Design review of the part built by this model. Coordinates are the model's own, in mm. Face numbers are marked on the shaded views. A direction names the side the tool comes from. Give positions to 0.01 mm unless a question says otherwise; leave off trailing zeros. Order: outer loops, then holes, each group sorted by start corner. A loop starts at its lowest first (then second) coordinate and runs counter-clockwise, first axis right, second up. Notation, with made-up numbers: M 55,56 L 112,56 A22 ccw 112,85 Z; hole C 22,78 d6. An arc over 180 degrees is marked long. Put each result on its own line as item: value. Start each with the question number.
from build123d import *

# Parameters (mm, degrees)
F1_DEPTH = 1180
F3_W     = 150
F3_H     = 125
F3_R     = 6
F4_DEPTH = 10
F7_W     = 150
F7_H     = 125
F7_R     = 6
F8_DEPTH = 10


with BuildPart() as f1:
    # F0 (on Front) → F1 (new body)
    with BuildSketch(Plane.XZ):
        with BuildLine():
            ThreePointArc((50, 45), (48.5355339059, 48.5355339059), (45, 50))
            Line((45, 50), (-45, 50))
            ThreePointArc((-45, 50), (-48.5355339059, 48.5355339059), (-50, 45))
            Line((-50, 45), (-50, -45))
            ThreePointArc((-50, -45), (-48.5355339059, -48.5355339059), (-45, -50))
            Line((-45, -50), (45, -50))
            ThreePointArc((45, -50), (48.5355339059, -48.5355339059), (50, -45))
            Line((50, -45), (50, 45))
        make_face()
        with BuildLine():
            ThreePointArc((-47, 45), (-46.4142135624, 46.4142135624), (-45, 47))
            Line((-45, 47), (45, 47))
            ThreePointArc((45, 47), (46.4142135624, 46.4142135624), (47, 45))
            Line((47, 45), (47, -45))
            ThreePointArc((47, -45), (46.4142135624, -46.4142135624), (45, -47))
            Line((45, -47), (-45, -47))
            ThreePointArc((-45, -47), (-46.4142135624, -46.4142135624), (-47, -45))
            Line((-47, -45), (-47, 45))
        make_face(mode=Mode.SUBTRACT)
    extrude(amount=-F1_DEPTH)


with BuildPart() as f4:
    # F3 (on offset) → F4 (new body)
    with BuildSketch(Plane.XZ.offset(10)):
        with Locations((0, 12.5)):
            Rectangle(F3_W, F3_H)
        with Locations((-62.5, -37.5)):
            Circle(F3_R, mode=Mode.SUBTRACT)
        with Locations((-62.5, 7.5)):
            Circle(F3_R, mode=Mode.SUBTRACT)
        with Locations((62.5, -37.5)):
            Circle(F3_R, mode=Mode.SUBTRACT)
        with Locations((62.5, 7.5)):
            Circle(F3_R, mode=Mode.SUBTRACT)
        with Locations((-62.5, 62.5)):
            Circle(F3_R, mode=Mode.SUBTRACT)
        with Locations((0, 62.5)):
            Circle(F3_R, mode=Mode.SUBTRACT)
        with Locations((62.5, 62.5)):
            Circle(F3_R, mode=Mode.SUBTRACT)
    extrude(amount=-F4_DEPTH)


with BuildPart() as f1_1:
    add(f1.part)

    # F5: union F4
    add(f4.part)

    # F7 (on offset) → F8 (join)
    with BuildSketch(Plane(origin=(0, 1190, 0), x_dir=(-1, 0, 0), z_dir=(0, 1, 0))):
        with Locations((0, 12.5)):
            Rectangle(F7_W, F7_H)
        with Locations((-62.5, -37.5)):
            Circle(F7_R, mode=Mode.SUBTRACT)
        with Locations((-62.5, 7.5)):
            Circle(F7_R, mode=Mode.SUBTRACT)
        with Locations((62.5, -37.5)):
            Circle(F7_R, mode=Mode.SUBTRACT)
        with Locations((62.5, 7.5)):
            Circle(F7_R, mode=Mode.SUBTRACT)
        with Locations((-62.5, 62.5)):
            Circle(F7_R, mode=Mode.SUBTRACT)
        with Locations((0, 62.5)):
            Circle(F7_R, mode=Mode.SUBTRACT)
        with Locations((62.5, 62.5)):
            Circle(F7_R, mode=Mode.SUBTRACT)
    extrude(amount=-F8_DEPTH)


solid = f1_1.part
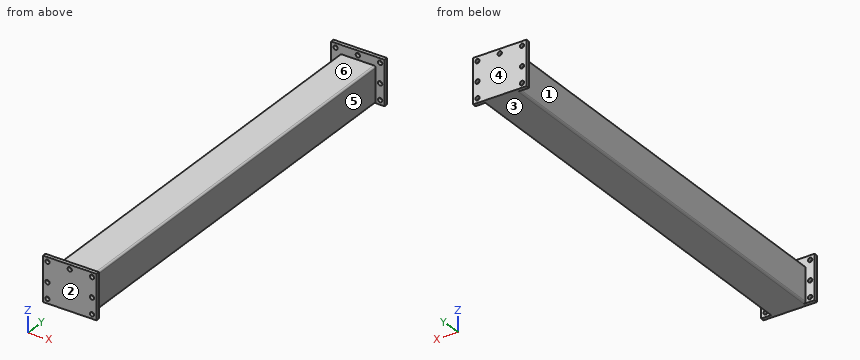
1. The part is to be moulded in two halves that separate along Y. For the marked faces 1, 2 and 3, say which applies: +Y half, -Y half, draft (parallel to the pull), parting line (faces both ways), or undercut.
2. Consider section B-B on y = 882. Give the boundary of the cut face in (x, z).
3. Insertion check: pin 1 (3 mm diameter, centred on y = 768.5, z = -18, fed in from -X); pin 2 (7 mm diameter, centred on x = 62.5, z = 7.5, fed in from -Y); pin 3 (3 mm diameter, centred on x = 31.5, y = 459, fed in from +Z); pin 4 (2 mm diameter, centred on y = 389.5, z = 46.5, fed in from +X). Each pin has a flat end and moves straight along its axis. Give the tip position at first contact, or say it passes through.
4. Consider section A-A on z = -10. Give the boundary of the cut face in (x, y).
5. Machinability: for the marked faces 4, 5 and 6, which of the approach directions +Z, -Z, +X, -X, +Y, -Y give a long, thin tool a straight path to every point of the face, cutting with its end or side? Answer none if there is none.
6. To check wall thickness, follow probe 1 along Z at (x, y) = (-62.5, 1186.5); probe 2 along X at (y, z) = (507, -3.5); probe 3 along Y at (x, z) = (-25.5, 40). State the ranges of each line that lie inside material, in increasing order.
Returned:
1. face 1: undercut
1. face 2: -Y half
1. face 3: draft
2. outline: M -50,-45 A5 ccw -45,-50 L 45,-50 A5 ccw 50,-45 L 50,45 A5 ccw 45,50 L -45,50 A5 ccw -50,45 Z; hole M -47,-45 A2 ccw -45,-47 L 45,-47 A2 ccw 47,-45 L 47,45 A2 ccw 45,47 L -45,47 A2 ccw -47,45 Z
3. pin 1: stops at x = -50
3. pin 2: passes through
3. pin 3: stops at z = 50
3. pin 4: stops at x = 49.97
4. outline: M -75,-10 L 75,-10 L 75,0 L 50,0 L 50,1180 L 75,1180 L 75,1190 L -75,1190 L -75,1180 L -50,1180 L -50,0 L -75,0 Z; hole M -47,0 L 47,0 L 47,1180 L -47,1180 Z
5. face 4: +Z, -Z, +X, -X, +Y
5. face 5: +Z, -Z, +X
5. face 6: +Z, +X, -X
6. probe 1: z = -50 to -43.5, -31.5 to 1.5, 13.5 to 56.5, 68.5 to 75
6. probe 2: x = -50 to -47, 47 to 50
6. probe 3: y = -10 to 0, 1180 to 1190
